Geometry: final body of the model. Coordinates: model frame, mm. A direction names the side the tool comes from. Give positions to 0.01 mm unless a question says otherwise; leave off trailing zeros. Write each loop counter-clockwise with the first axis right and the second up, starting at its lowest first coordinate (ties: lowest second). Pieces come first, ordered by that corner, then holes.
Q1. Cut plane C-C on x = 0. Return the cut outline in (y, z).
Q2. Pin query (flat end, axial travel): pin 1 (1 mm diameter, centred on y = -0.5, z = 12, fed in from +X); pin 2 (4 mm diameter, centred on y = -4, z = -12, fed in from +X); pin 3 (0.7 mm diameter, centred on x = -4, z = 14.5, fed in from +Y); pin 4 (1.9 mm diameter, centred on x = 0, z = 0, fed in from -Y). Return the tip coordinate at first contact, or that it passes through.
Q3. Draft query along Z for faces 1 (the face through (0, 6.25, 15)), 2 (the face through (2.685, 0.334, 0.596)), 3 (the face through (15.62, 0.33, 3.47)). Return one class per face: pulls with the +Z half, pulls with the -Z half, needs draft (parallel to the pull), parting line crosses it, or undercut.
Q4. Cut plane A-A on y = 4. Return the cut outline in (x, z).
Q5. Cut plane B-B on z = 0. Return the cut outline in (x, y).
Q6. Line query: L1, parallel to X at y = 2, z = 0; L2, parallel to Y at x = 11.5, z = -5.5; L3, parallel to Z at x = -8, y = 1.5. Output: solid intervals per line, ascending.
Q7. Reachability of faces 4 (the face through (0, 6.25, -2)), 5 (the face through (2.1, 5, 15)), 6 (the face through (0, -5.75, -3)) from +Z, -Z, +X, -X, +Y, -Y: full face, straight path, thin tool, end or side. Return the list, or none.
```python
from build123d import *

# Parameters (mm, degrees)
CUT_EXTRUDE1_START = 10
SKETCH2_W          = 2.8
SKETCH2_H          = 2.8
CUT_EXTRUDE1_DEPTH = 10


with BuildPart() as part:
    # Sketch1 → Revolve1 (revolve)
    with BuildSketch(Plane.XY, mode=Mode.PRIVATE) as revolve1_sk:
        Polygon((-14.5, 6.25), (-14.5, -4.75), (-13.5, -5.75), (-2.75, -5.75), (-2.75, 6.25), (-1.6, 6.25), (-1.6, -6.75), (-15.002979439, -6.75), (-16, -5.752979439), (-16, 6.25), align=None)
    revolve(revolve1_sk.sketch.rotate(Axis((0, 0, 0), (0, 1, 0)), 270), axis=Axis((0, 0, 0), (0, 1, 0)))

    # Sketch2 → Cut-Extrude1 (cut)
    with BuildSketch(Plane.XY.offset(CUT_EXTRUDE1_START)):
        with Locations((-3.5, 4.85)):
            Rectangle(SKETCH2_W, SKETCH2_H)
        with Locations((3.5, 4.85)):
            Rectangle(SKETCH2_W, SKETCH2_H)
    extrude(amount=CUT_EXTRUDE1_DEPTH, mode=Mode.SUBTRACT)


solid = part.part
```
Data:
1. outline: (-6.75, -15) - (-5.75, -16) - (6.25, -16) - (6.25, -14.5) - (-4.75, -14.5) - (-5.75, -13.5) - (-5.75, -2.75) - (6.25, -2.75) - (6.25, -1.6) - (-6.75, -1.6) - close; (-6.75, 1.6) - (6.25, 1.6) - (6.25, 2.75) - (-5.75, 2.75) - (-5.75, 13.5) - (-4.75, 14.5) - (6.25, 14.5) - (6.25, 16) - (-5.75, 16) - (-6.75, 15) - close
2. pin 1: stops at x = 11.12
2. pin 2: stops at x = 12.49
2. pin 3: stops at y = 3.45
2. pin 4: passes through
3. face 1: needs draft
3. face 2: undercut
3. face 3: parting line crosses it
4. outline: (-4.9, 13.65) - (-4.9, 15.23) arc R16 ccw (long way) to (4.9, 15.23) - (4.9, 13.65) arc R14.5 cw (long way) to start; circle Ø5.5 at (0, 0); (-2.1, 14.35) arc R14.5 cw to (2.1, 14.35) - (2.1, 15.86) arc R16 ccw to (-2.1, 15.86) - close; hole circle Ø3.2 at (0, 0)
5. outline: (-16, -5.75) - (-15, -6.75) - (-1.6, -6.75) - (-1.6, 6.25) - (-2.75, 6.25) - (-2.75, -5.75) - (-13.5, -5.75) - (-14.5, -4.75) - (-14.5, 6.25) - (-16, 6.25) - close; (1.6, -6.75) - (15, -6.75) - (16, -5.75) - (16, 6.25) - (14.5, 6.25) - (14.5, -4.75) - (13.5, -5.75) - (2.75, -5.75) - (2.75, 6.25) - (1.6, 6.25) - close
6. L1: x = -16 to -14.5, -2.75 to -1.6, 1.6 to 2.75, 14.5 to 16
6. L2: y = -6.75 to -5.75
6. L3: z = -13.86 to -12.09, 12.09 to 13.86
7. face 4: +Z, -Z, +X, -X, +Y
7. face 5: +Z, +Y
7. face 6: +Y
